from build123d import *

# Parameters (mm, degrees)
F0_W     = 12
F0_H     = 6
F1_DEPTH = 50
F2_R     = 5.99999
F4_DEPTH = 25
F6_DEPTH = 60
F7_SIZE  = 2
F8_SIZE  = 1


# Not quite as in the source:
# - a fillet or chamfer is up to 0.001 mm smaller than in the source, because OpenCascade refuses the exact size


with BuildPart() as f1:
    # F0 (on Front) → F1 (new body)
    with BuildSketch(Plane.XZ):
        Polygon((0, 27), (0, 0), (20, 0), (23, 0), (35, 0), (40, 0), (40, 6), (5, 6), (5, 21), (40, 21), (40, 27), align=None)
        with Locations((29, -3)):
            Rectangle(F0_W, F0_H)
    extrude(amount=F1_DEPTH)

    # F2 (radius 6 in the source; OpenCascade refuses exactly that, so slightly less here)
    f2_edges = [f1.edges().sort_by_distance(p)[0] for p in [
        (23, -25, -6),
        (35, -25, -6),
    ]]
    fillet(f2_edges, radius=F2_R)

    # F3 (on face) → F4 (cut)
    with BuildSketch(Plane.XY.offset(6)):
        Polygon((40, -35), (40, -25), (40, -15), (5, -15), (5, -35), align=None)
    extrude(amount=-F4_DEPTH, mode=Mode.SUBTRACT)

    # F5 (on face) → F6 (cut)
    with BuildSketch(Plane.XZ.offset(50)):
        with BuildLine():
            ThreePointArc((29, -2.5), (30.767766953, -1.767766953), (31.5, 0))
            ThreePointArc((31.5, 0), (27.232233047, 1.767766953), (29, -2.5))
        make_face()
    extrude(amount=-F6_DEPTH, mode=Mode.SUBTRACT)

    # F7
    f7_edges = [f1.edges().sort_by_distance(p)[0] for p in [
        (0, -25, 27),
        (40, -25, 27),
        (0, -25, 0),
        (40, -42.5, 0),
        (40, -7.5, 0),
    ]]
    chamfer(f7_edges, length=F7_SIZE)

    # F8
    f8_edges = [f1.edges().sort_by_distance(p)[0] for p in [
        (40, -42.5, 6),
        (40, -7.5, 6),
        (40, -25, 21),
    ]]
    chamfer(f8_edges, length=F8_SIZE)


solid = f1.part
Build history of the part. All positions in model axes, mm. A direction names the side the tool comes from. Round coordinates to 2 decimals unless told otherwise and drop trailing zeros. Loops run counter-clockwise (first coordinate to the right, second up) from the corner with the lowest first, then second, coordinate; pieces in that order, holes last. Notation, with made-up numbers: (82.5, 73) -> (136.5, 73) arc R17 ccw to (136.5, 78) -> close; hole circle Ø6 at (57, 5.25). An arc over 180 degrees is marked (long way). Answer in a Markdown table with one row per item.
Item 1: Pin check, flat tips, straight feed: pin 1 (3 mm diameter, centred on x = 16, y = -30.5, fed in from -Z); pin 2 (9.5 mm diameter, centred on x = 30, z = 1.5, fed in from -Y); pin 3 (23 mm diameter, centred on x = 15, y = -29.5, fed in from -Z); pin 4 (6.5 mm diameter, centred on y = -31.5, z = 9, fed in from +X). Stop position of each tip, or through.
Answers below:
| item | result |
|---|---|
| pin 1 | stops at z = 21 |
| pin 2 | stops at y = -50 |
| pin 3 | stops at z = -4.56 |
| pin 4 | stops at x = 5 |
Item 2: Mould opens along Y. For faces 5 (the flat face through (22, -35, 1)), 6 (the flat face through (1, -25, 26)), 7 (the flat face through (20, -50, 22)) say: +Y half, -Y half, draft (parallel to the pull), parting line (faces both ways), or undercut.
Answers below:
| item | result |
|---|---|
| face 5 | undercut |
| face 6 | draft |
| face 7 | -Y half |
Item 3: Drill centre lines: L1, parallel to Z at x = 29, y = -39.5; L2, parallel to Y at x = 20.5, z = 1; L3, parallel to Z at x = 29.5, y = -2.5. Where is each one in solid material? Low to high. Write a range as [from, to].
Answers below:
| item | result |
|---|---|
| L1 | z = [-6, -2.5], [2.5, 6], [21, 27] |
| L2 | y = [-50, -35], [-15, 0] |
| L3 | z = [-5.98, -2.45], [2.45, 6], [21, 27] |
Item 4: Which spindle directions (+Z, -Z, +X, -X, +Y, -Y) get a long thin tool onto all of the face, cutting with end or side? Do faces 1 (the flat face through (3, -25, 0)), 2 (the flat face through (22, -7, 6)), 3 (the flat face through (36, -42, 0)), 4 (the flat face through (5, -25, 13)). Say none if no direction does.
Answers below:
| item | result |
|---|---|
| face 1 | -Z, -X, +Y, -Y |
| face 2 | +X, +Y, -Y |
| face 3 | -Z, +X, +Y, -Y |
| face 4 | +X |
Item 5: Saw through at D-D (y = -19). Write the cut outline in (x, z), and give its area (4 significant figures).
Answers below:
| item | result |
|---|---|
| outline | (0, 2) -> (2, 0) -> (5, 0) -> (5, 21) -> (39, 21) -> (40, 22) -> (40, 25) -> (38, 27) -> (2, 27) -> (0, 25) -> close |
| area | 338.5 mm² |
Item 6: Saw through at C-C (z = -1.5). Write the cut outline in (x, y).
Answers below:
| item | result |
|---|---|
| outline | (23.19, -50) -> (27, -50) -> (27, -35) -> (23.19, -35) -> close; (23.19, -15) -> (27, -15) -> (27, 0) -> (23.19, 0) -> close; (31, -50) -> (34.81, -50) -> (34.81, -35) -> (31, -35) -> close; (31, -15) -> (34.81, -15) -> (34.81, 0) -> (31, 0) -> close |
Item 7: Saw through at B-B (x = 9.5). Write the cut outline in (y, z), and give its area (3 significant figures).
Answers below:
| item | result |
|---|---|
| outline | (-50, 0) -> (-35, 0) -> (-35, 6) -> (-50, 6) -> close; (-50, 21) -> (0, 21) -> (0, 27) -> (-50, 27) -> close; (-15, 0) -> (0, 0) -> (0, 6) -> (-15, 6) -> close |
| area | 480 mm² |
